Here's how the part is built. I have some questions about the finished solid (model axes, mm). A direction names the side the tool comes from. Round coordinates to 2 decimals unless told otherwise and drop trailing zeros. Order: outer loops, then holes, each group sorted by start corner. A loop starts at its lowest first (then second) coordinate and runs counter-clockwise, first axis right, second up. Notation, with made-up numbers: (61, 4) - (113, 4) arc R17 ccw to (113, 12) - close; hole circle Ø9 at (27.5, -32). An arc over 180 degrees is marked (long way). Answer as a JSON object with one key per item and string values.
Autodesk Inventor part; units mm, degrees
ref_plane "YZ Plane" through (0, 0, 0) normal (1, 0, 0) x (0, 1, 0)
ref_plane "XZ Plane" through (0, 0, 0) normal (0, 1, 0) x (-1, 0, 0)
ref_plane "XY Plane" through (0, 0, 0) normal (0, 0, 1) x (1, 0, 0)
sketch "Boceto1" plane through (0, 0, 0) normal (0, 1, 0) x (-1, 0, 0)
  line L0 (50, 50) -> (-50, 50)
  line L1 (-50, 50) -> (-50, -50)
  line L2 (-50, -50) -> (50, -50)
  line L3 (50, -50) -> (50, 50)
  line L4 (50, 50) -> (-50, -50) construction
  line L5 (-50, 50) -> (50, -50) construction
  point P0 (0, 0)
  dimension "d0" = 100
  dimension "d1" = 100
extrude "Extrusión1" add sketch "Boceto1" along normal blind 10
sketch "Boceto2" plane through (0, 10, 0) normal (0, 1, 0) x (1, 0, 0)
  line L0 (-15, 35) -> (15, 35)
  line L1 (15, 35) -> (15, -35)
  line L2 (15, -35) -> (-15, -35)
  line L3 (-15, -35) -> (-15, 35)
  line L4 (-15, 35) -> (15, -35) construction
  line L5 (15, 35) -> (-15, -35) construction
  point P0 (0, 0)
  dimension "d4" = 70
  dimension "d5" = 30
extrude "Extrusión2" add sketch "Boceto2" along normal blind 80
sketch "Boceto3" plane through (-15, 10, -35) normal (-1, 0, 0) x (0, 0, 1)
  circle A0 centre (35, 55) radius 8.5
  line L0 (0, 0) -> (0, 80)
  line L1 (0, 80) -> (70, 80)
  point P0 (35, -10)
  dimension "d8" = 17
  dimension "d9" = 35
  dimension "d10" = 25
extrude "Extrusión3" cut sketch "Boceto3" along normal mid plane 80
fillet "Empalme1" radius 35 1 edges at (0, 90, -35)
fillet "Empalme2" radius 35 1 edges at (0, 90, 35)
properties part number "02_10 Soporte01" material "Acero ASTM A36"
1. Imagine slicing it at D-D (z = 26). List the corners of the cut face in (x, y) for me, plus the area to 3 significant figures.
Responses:
{"outline": "(-50, 0) - (50, 0) - (50, 10) - (15, 10) - (15, 78.43) - (-15, 78.43) - (-15, 10) - (-50, 10) - close", "area": "3,050 mm2"}
2. If I drill on L1, parallel to Y at x = -1, z = 0; L2, parallel to Y at x = -36.5, z = -22; L3, parallel to X at y = 47.5, z = -2, over which ranges is the centre line in solid material (lowest first)? Write a range as [from, to].
Responses:
{"L1": "[0, 56.5], [73.5, 90]", "L2": "[0, 10]", "L3": "[-15, 15]"}
3. Thinking about a two-plate mould opening in Z: for faces 6 (the face through (-1, 5, 50)), 7 (the face through (-50, 5, -1)), 8 (the face through (-0.21, 56.7, -1.84)), which applies, pulls with the +Z half, pulls with the -Z half, needs draft (parallel to the pull), parting line crosses it, or undercut?
Responses:
{"face 6": "pulls with the +Z half", "face 7": "needs draft", "face 8": "undercut"}
4. Imagine slicing it at B-B (z = -36.5). List the corners of the cut face in (x, y) for me, plus the area to 3 significant figures.
Responses:
{"outline": "(-50, 0) - (50, 0) - (50, 10) - (-50, 10) - close", "area": "1,000 mm2"}
5. For faces 1 (the face through (0, 32, -35)), 2 (the face through (0, 32, 35)), 3 (the face through (50, 5, 1)), 4 (the face through (15, 49, 0)), 5 (the face through (-15, 49, 0)), which set-ups out of +Z, -Z, +X, -X, +Y, -Y let a thin tool reach every point of the face, with its end or its side?
Responses:
{"face 1": "-Z, +X, -X, +Y", "face 2": "+Z, +X, -X, +Y", "face 3": "+Z, -Z, +X, +Y, -Y", "face 4": "+Z, -Z, +X, +Y", "face 5": "+Z, -Z, -X, +Y"}
6. Imagine slicing it at A-A (y = 65). List the corners of the cut face in (x, z) for me.
Responses:
{"outline": "(-15, -33.54) - (15, -33.54) - (15, -8.5) - (-15, -8.5) - close; (-15, 8.5) - (15, 8.5) - (15, 33.54) - (-15, 33.54) - close"}
7. Imagine slicing it at C-C (y = 38). List the corners of the cut face in (x, z) for me.
Responses:
{"outline": "(-15, -35) - (15, -35) - (15, 35) - (-15, 35) - close"}
8. For P1, Ø1, axis at y = 22, z = -16.5, coming from the +X side; P2, Ø9, axis at x = 3, y = 21.5, coming from the -Z side; P3, Ø15, axis at x = -7.5, y = 30, coming from the +Z side, each with a flat end and sliding along its axis, tell me the tip position at first contact or that it passes through.
Responses:
{"P1": "x = 15", "P2": "z = -35", "P3": "z = 35"}
